Here's how the part is built. I have some questions about the finished solid (model axes, mm). A direction names the side the tool comes from. Round coordinates to 2 decimals unless told otherwise and drop trailing zeros. Write each loop counter-clockwise with the first axis right and the second up, starting at its lowest first coordinate (ties: lowest second). Pieces come first, ordered by that corner, then holes. Notation, with made-up numbers: (1.5, -13.75) -> (44.5, -13.75) arc R25 ccw to (44.5, 2.25) -> close; hole circle Ø7 at (-21, 78). An arc over 180 degrees is marked (long way). Answer as CSV lines item,"result".
```python
from build123d import *

# Parameters (mm, degrees)
F0_W     = 20
F0_H     = 20
F0_W_2   = 320
F1_DEPTH = 150
F0_H_2   = 210
F2_DEPTH = 140
F3_DEPTH = 25


with BuildPart() as f1:
    # F0 (on Top) → F1 (new body)
    with BuildSketch(Plane.XY):
        with Locations((-170, -115)):
            Rectangle(F0_W, F0_H)
        with Locations((0, -115)):
            Rectangle(F0_W_2, F0_H)
        with Locations((170, -115)):
            Rectangle(F0_W, F0_H)
    extrude(amount=F1_DEPTH)

    # F0 (on Top) → F2 (join)
    with BuildSketch(Plane.XY):
        with Locations((-170, 0)):
            Rectangle(F0_W, F0_H_2)
        with Locations((-170, 115)):
            Rectangle(F0_W, F0_H)
        with Locations((0, 115)):
            Rectangle(F0_W_2, F0_H)
        with Locations((170, 115)):
            Rectangle(F0_W, F0_H)
        with Locations((170, 0)):
            Rectangle(F0_W, F0_H_2)
    extrude(amount=F2_DEPTH)

    # F0 (on Top) → F3 (join)
    with BuildSketch(Plane.XY):
        Rectangle(F0_W_2, F0_H_2)
    extrude(amount=F3_DEPTH)


solid = f1.part
```
1. Suppose I cut it at B-B on z = 40.5. Please give me the cut outline in (x, y), and give its area (3 significant figures).
Numbers:
outline,"(-180, -125) -> (180, -125) -> (180, 125) -> (-180, 125) -> close; hole (-160, -105) -> (160, -105) -> (160, 105) -> (-160, 105) -> close"
area,"22,800 mm^2"
2. If I drill on line 1 (Y direction, x = 40, z = 31); line 2 (X direction, y = -103.5, z = 84); line 3 (Z direction, x = -138, y = 18.5), over which ranges is the centre line in solid material (lowest first)?
Numbers:
line 1,"y = -125 to -105, 105 to 125"
line 2,"x = -180 to -160, 160 to 180"
line 3,"z = 0 to 25"
3. Suppose I cut it at A-A on y = 5. Please give me the cut outline in (x, z).
Numbers:
outline,"(-180, 0) -> (180, 0) -> (180, 140) -> (160, 140) -> (160, 25) -> (-160, 25) -> (-160, 140) -> (-180, 140) -> close"
4. If we mould it in two halves opening along Y, with no side actions, what happens to faces 4 (the face through (-3, -125, 74)), 5 (the face through (160, -1, 82)), 6 (the face through (-160, -1, 82)), 7 (the face through (3, 125, 69))? For each: released by +Y, released by -Y, zero draft, split by the parting line, or undercut.
Numbers:
face 4,"released by -Y"
face 5,"undercut"
face 6,"undercut"
face 7,"released by +Y"
5. Suppose I cut it at C-C on x = 126.5. Please give me the cut outline in (y, z).
Numbers:
outline,"(-125, 0) -> (125, 0) -> (125, 140) -> (105, 140) -> (105, 25) -> (-105, 25) -> (-105, 150) -> (-125, 150) -> close"
6. On a 3-axis mill with a long thin cutter (end or side, diameter ignored), from which of +Z, -Z, +X, -X, +Y, -Y can I reach the whole of each face in a straight line? I mean faces 1 (the face through (-3, 2, 0)), 2 (the face through (-41, 113, 140)), 3 (the face through (-2, 1, 25)). Say none if no direction works.
Numbers:
face 1,"-Z, +X, -X, +Y, -Y"
face 2,"+Z, +X, -X, +Y"
face 3,"+Z"
